Here's how the part is built. I have some questions about the finished solid (model axes, mm). Give positions to 0.01 mm unless a question says otherwise; leave off trailing zeros. Write each loop counter-clockwise with the first axis right and the second up, starting at its lowest first coordinate (ties: lowest second). Pieces come first, ordered by that corner, then holes. Notation, with made-up numbers: (9.5, 25) - (16.5, 25) arc R27 ccw to (16.5, 56) - close; hole circle Ø7 at (-36, -15). An arc over 180 degrees is marked (long way). Use a Markdown table: item, result.
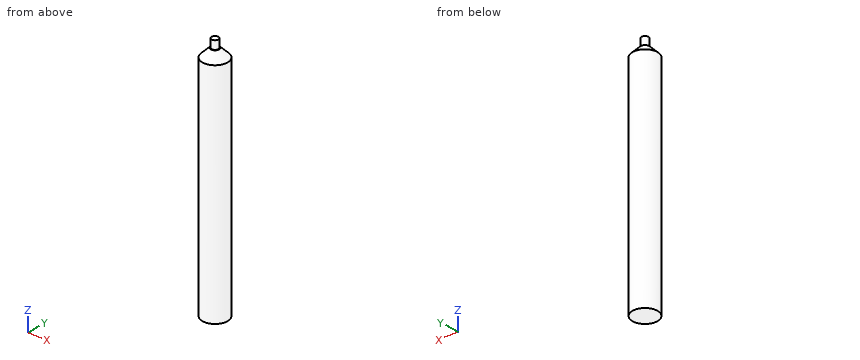
Autodesk Inventor part; units mm, degrees
ref_plane "YZ Plane" through (0, 0, 0) normal (1, 0, 0) x (0, 1, 0)
ref_plane "XZ Plane" through (0, 0, 0) normal (0, 1, 0) x (-1, 0, 0)
ref_plane "XY Plane" through (0, 0, 0) normal (0, 0, 1) x (1, 0, 0)
sketch "Sketch2" plane through (0, 0, 0) normal (0, 0, 1) x (-1, 0, 0)
  circle A0 centre (0, 0) radius 7.5
  dimension "d0" = 15
extrude "Extrusion1" add sketch "Sketch2" along normal blind 140
sketch "Sketch3" plane through (0, 0, 140) normal (0, 0, 1) x (1, 0, 0)
  circle A0 centre (0, 0) radius 2
  dimension "d3" = 4
extrude "Extrusion2" add sketch "Sketch3" along normal blind 5
chamfer "Chamfer1" distance 5 angle 45 1 edges at (7.5, 0, 140)
properties part number "Marcador"
Item 1: If we section it at A-A, the plane x = 0: Write out the boundary of the cut face in (y, z), plus the area to 4 significant figures.
Values:
| item | result |
|---|---|
| outline | (-7.5, 0) - (7.5, 0) - (7.5, 135) - (2.5, 140) - (2, 140) - (2, 145) - (-2, 145) - (-2, 140) - (-2.5, 140) - (-7.5, 135) - close |
| area | 2,095 mm2 |
Item 2: I need wall thicknesses on line 1 along Z through (x, y) = (7, -0.75); line 2 along Y through (x, z) = (-4.5, 135.5); line 3 along X through (y, z) = (-5.75, 34). Which ranges of each line are inside material? Lowest first, please. Write a range as [from, to].
Values:
| item | result |
|---|---|
| line 1 | z = [0, 135.46] |
| line 2 | y = [-5.36, 5.36] |
| line 3 | x = [-4.82, 4.82] |
Item 3: If we section it at C-C, the plane z = 120.5: Write out the boundary of the cut face in (x, y).
Values:
| item | result |
|---|---|
| outline | circle Ø15 at (0, 0) |
Item 4: Will these pins go through, and if not, where does the flat tip stop? pin 1 Ø2 at (x, z) = (3, 116) entering from +Y; pin 2 Ø2 at (x, z) = (-1.5, 35.5) entering from -Y; pin 3 Ø8 at (y, z) = (5.5, 69.5) entering from +X.
Values:
| item | result |
|---|---|
| pin 1 | stops at y = 7.23 |
| pin 2 | stops at y = -7.48 |
| pin 3 | stops at x = 7.35 |
